```python
from build123d import *

# Parameters (mm, degrees)
SKETCH_1_W          = 10
SKETCH_1_H          = 10
SKETCH_1_W_2        = 8
SKETCH_1_H_2        = 8
EXTRUDE_1_DEPTH     = 80
SKETCH_2_R          = 3
CUT_EXTRUDE_1_DEPTH = 81.777472107
SKETCH_3_R          = 3
CUT_EXTRUDE_2_DEPTH = 10
SKETCH_4_R          = 1.6
CUT_EXTRUDE_3_DEPTH = 10
SKETCH_5_R          = 1.6
CUT_EXTRUDE_4_DEPTH = 81.777472107
SKETCH_6_W          = 10
SKETCH_6_H          = 45
CUT_EXTRUDE_5_DEPTH = 10
SKETCH_7_R          = 3
CUT_EXTRUDE_6_DEPTH = 2


with BuildPart() as part:
    # ｽｹｯﾁ1 → ﾎﾞｽ - 押し出し1 (new body)
    with BuildSketch(Plane.XY):
        Rectangle(SKETCH_1_W, SKETCH_1_H)
        Rectangle(SKETCH_1_W_2, SKETCH_1_H_2, mode=Mode.SUBTRACT)
    extrude(amount=EXTRUDE_1_DEPTH)

    # ｽｹｯﾁ2 → ｶｯﾄ - 押し出し1 (cut, through all)
    with BuildSketch(Plane.ZY.offset(5)):
        with Locations((5, 0)):
            Circle(SKETCH_2_R)
        with Locations((75, 0)):
            Circle(SKETCH_2_R)
    extrude(amount=-CUT_EXTRUDE_1_DEPTH, mode=Mode.SUBTRACT)

    # ｽｹｯﾁ3 → ｶｯﾄ - 押し出し2 (cut)
    with BuildSketch(Plane(origin=(0, 5, 0), x_dir=(1, 0, 0), z_dir=(0, 1, 0))):
        with Locations(Location((0, -65, 0), (0, 0, 270))):
            Circle(SKETCH_3_R)
        with Locations(Location((0, -15, 0), (0, 0, 270))):
            Circle(SKETCH_3_R)
    extrude(amount=-CUT_EXTRUDE_2_DEPTH, mode=Mode.SUBTRACT)

    # ｽｹｯﾁ4 → ｶｯﾄ - 押し出し3 (cut)
    with BuildSketch(Plane(origin=(0, 5, 0), x_dir=(1, 0, 0), z_dir=(0, 1, 0))):
        with Locations(Location((0, -30, 0), (0, 0, 270))):
            Circle(SKETCH_4_R)
        with Locations(Location((0, -50, 0), (0, 0, 270))):
            Circle(SKETCH_4_R)
    extrude(amount=-CUT_EXTRUDE_3_DEPTH, mode=Mode.SUBTRACT)

    # ｽｹｯﾁ5 → ｶｯﾄ - 押し出し4 (cut, through all)
    with BuildSketch(Plane.ZY.offset(5)):
        with Locations((25, 0)):
            Circle(SKETCH_5_R)
        with Locations((55, 0)):
            Circle(SKETCH_5_R)
    extrude(amount=-CUT_EXTRUDE_4_DEPTH, mode=Mode.SUBTRACT)

    # ｽｹｯﾁ6 → ｶｯﾄ - 押し出し5 (cut)
    with BuildSketch(Plane(origin=(0, 5, 0), x_dir=(1, 0, 0), z_dir=(0, 1, 0))):
        with Locations((0, -57.5)):
            Rectangle(SKETCH_6_W, SKETCH_6_H)
    extrude(amount=-CUT_EXTRUDE_5_DEPTH, mode=Mode.SUBTRACT)

    # ｽｹｯﾁ7 → ｶｯﾄ - 押し出し6 (cut)
    with BuildSketch(Plane(origin=(0, 5, 0), x_dir=(1, 0, 0), z_dir=(0, 1, 0))):
        with Locations(Location((0, -30, 0), (0, 0, 270))):
            Circle(SKETCH_7_R)
    extrude(amount=-CUT_EXTRUDE_6_DEPTH, mode=Mode.SUBTRACT)


solid = part.part
```
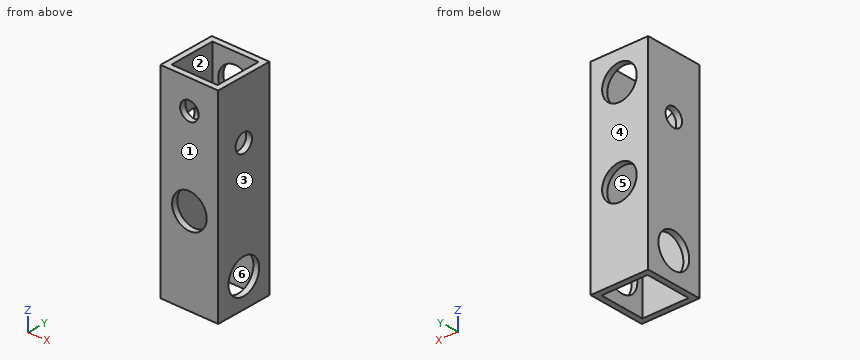
Here's how the part is built. I have some questions about the finished solid (model axes, mm). Face numbers are marked on the shaded views. A direction names the side the tool comes from. Coordinates: 2 decimals unless noted, no trailing zeros. Order: outer loops, then holes, each group sorted by start corner. A loop starts at its lowest first (then second) coordinate and runs counter-clockwise, first axis right, second up.
Item 1: If we section it at A-A, the plane z = 30: List the corners of the cut face in (x, y) for me.
Response values:
outline: (-5, -5) - (-1.6, -5) - (-1.6, -4) - (-4, -4) - (-4, 4) - (-3, 4) - (-3, 5) - (-5, 5) - close; (1.6, -5) - (5, -5) - (5, 5) - (3, 5) - (3, 4) - (4, 4) - (4, -4) - (1.6, -4) - close
Item 2: If we section it at C-C, the plane z = 10: List the corners of the cut face in (x, y) for me.
Response values:
outline: (-5, -5) - (5, -5) - (5, 5) - (-5, 5) - close; hole (-4, -4) - (4, -4) - (4, 4) - (-4, 4) - close
Item 3: I'm going to push a flat-ended pin straight in: pin 1 Ø1.9 at (y, z) = (0, 25) entering from +X. Where does the tip first touch, or does it pass through?
Response values:
pin 1: passes through
Item 4: I need wall thicknesses on probe 1 along Y at (x, z) = (0.25, 6.5); probe 2 along Y at (x, z) = (-4.6, 5). Which ranges of each line are inside material? Lowest first, please.
Response values:
probe 1: y = -5 to -4, 4 to 5
probe 2: y = -5 to -3, 3 to 5
Item 5: Thinking about a two-plate mould opening in X: for the marked faces 3, 4, 5 and 6, which applies, pulls with the +X half, pulls with the -X half, needs draft (parallel to the pull), parting line crosses it, or undercut?
Response values:
face 3: pulls with the +X half
face 4: needs draft
face 5: undercut
face 6: undercut
Item 6: If we section it at D-D, the plane y = -0.5: List the corners of the cut face in (x, z) for me.
Response values:
outline: (-5, 0) - (-4, 0) - (-4, 2.04) - (-5, 2.04) - close; (-5, 7.96) - (-4, 7.96) - (-4, 23.48) - (-5, 23.48) - close; (-5, 26.52) - (-4, 26.52) - (-4, 35) - (-5, 35) - close; (4, 0) - (5, 0) - (5, 2.04) - (4, 2.04) - close; (4, 7.96) - (5, 7.96) - (5, 23.48) - (4, 23.48) - close; (4, 26.52) - (5, 26.52) - (5, 35) - (4, 35) - close
Item 7: If we section it at B-B, the plane y = -2: List the corners of the cut face in (x, z) for me.
Response values:
outline: (-5, 0) - (-4, 0) - (-4, 2.76) - (-5, 2.76) - close; (-5, 7.24) - (-4, 7.24) - (-4, 35) - (-5, 35) - close; (4, 0) - (5, 0) - (5, 2.76) - (4, 2.76) - close; (4, 7.24) - (5, 7.24) - (5, 35) - (4, 35) - close
Item 8: Which directions (+Z, -Z, +X, -X, +Y, -Y) give clear straight access to the entire face, cutting with the end or side of a thin tool? Please do the marked faces 1 and 2.
Response values:
face 1: +Z, -Z, +X, -X, -Y
face 2: +Z, -Z
